from build123d import *

# Parameters (mm, degrees)
F0_W     = 800
F0_H     = 270
F1_DEPTH = 1060
F2_W     = 760
F2_H     = 50
F3_DEPTH = 20
F4_W     = 760
F4_H     = 310
F5_DEPTH = 260


with BuildPart() as f1:
    # F0 (on Top) → F1 (new body)
    with BuildSketch(Plane.XY):
        with Locations((143.156862, -15.404297)):
            Rectangle(F0_W, F0_H)
    extrude(amount=F1_DEPTH)

    # F2 (on face) → F3 (cut)
    with BuildSketch(Plane.XZ.offset(150.404297)):
        with Locations((143.156862, 25)):
            Rectangle(F2_W, F2_H)
    extrude(amount=-F3_DEPTH, mode=Mode.SUBTRACT)

    # F4 (on face) → F5 (cut)
    with BuildSketch(Plane.XZ.offset(150.404297)):
        with Locations((143.156862, 885)):
            Rectangle(F4_W, F4_H)
        with Locations((143.156862, 555)):
            Rectangle(F4_W, F4_H)
        with Locations((143.156862, 225)):
            Rectangle(F4_W, F4_H)
    extrude(amount=-F5_DEPTH, mode=Mode.SUBTRACT)


solid = f1.part
Read the model definition and answer for the solid it produces. Units are mm, in the model's axes. A direction names the side the tool comes from. Coordinates: 2 decimals unless noted, no trailing zeros. Order: outer loops, then holes, each group sorted by start corner. A loop starts at its lowest first (then second) coordinate and runs counter-clockwise, first axis right, second up. Notation, with made-up numbers: (-2, 78) -> (4, 78) arc R38 cw to (4, 116) -> close; hole circle Ø2 at (13.5, 65.5). An arc over 180 degrees is marked (long way). Answer as a JSON object with one key per item and string values.
1) Consider line 1 along Z through (x, y) = (265, -97); line 2 along X through (y, z) = (-49.5, 455); line 3 along Y through (x, z) = (-154, 342). Determine where each line is inside the solid, lowest interval first. Write a range as from..to.
Model answer:
{"line 1": "z = 0..70, 380..400, 710..730, 1040..1060", "line 2": "x = -256.84..-236.84, 523.16..543.16", "line 3": "y = 109.6..119.6"}
2) A tool of negligible diameter and unlimited length cuts with its end or side. For faces 4 (the face through (112, -150.404, 724)), 5 (the face through (138, -130.404, 25)), 6 (the face through (138, 109.596, 227)), from which of +Z, -Z, +X, -X, +Y, -Y can it reach the whole face along a straight path? Write none if from no direction.
Model answer:
{"face 4": "+Z, -Z, +X, -X, -Y", "face 5": "-Z, -Y", "face 6": "-Y"}
3) The mould has two halves that part along Z. Classify faces 1 (the face through (138, -22, 1040)), 2 (the face through (138, 16, 0)), 3 (the face through (543.157, -17, 523)): released by +Z, released by -Z, zero draft, split by the parting line, or undercut.
Model answer:
{"face 1": "undercut", "face 2": "released by -Z", "face 3": "zero draft"}
4) A cutting plane is placed at B-B, the plane y = -95.5. Determine the outline of the cut face in (x, z).
Model answer:
{"outline": "(-256.84, 0) -> (543.16, 0) -> (543.16, 1060) -> (-256.84, 1060) -> close; hole (-236.84, 70) -> (523.16, 70) -> (523.16, 380) -> (-236.84, 380) -> close; hole (-236.84, 400) -> (523.16, 400) -> (523.16, 710) -> (-236.84, 710) -> close; hole (-236.84, 730) -> (523.16, 730) -> (523.16, 1040) -> (-236.84, 1040) -> close"}
5) A cutting plane is placed at C-C, the plane x = -161. Determine the outline of the cut face in (y, z), plus the area to 3 significant figures.
Model answer:
{"outline": "(-150.4, 50) -> (-130.4, 50) -> (-130.4, 0) -> (119.6, 0) -> (119.6, 1060) -> (-150.4, 1060) -> (-150.4, 1040) -> (109.6, 1040) -> (109.6, 730) -> (-150.4, 730) -> (-150.4, 710) -> (109.6, 710) -> (109.6, 400) -> (-150.4, 400) -> (-150.4, 380) -> (109.6, 380) -> (109.6, 70) -> (-150.4, 70) -> close", "area": "43,400 mm²"}
6) Each of these flat-tipped pins is pushed along its axis until it touches: pin 1 (2 mm diameter, centred on x = 126.5, y = 39, fed in from -Z); pin 2 (10 mm diameter, centred on x = 75, y = -140, fed in from -Z); pin 3 (12 mm diameter, centred on x = -111.5, z = 455, fed in from -Y); pin 4 (25 mm diameter, centred on x = 279.5, z = 16.5, fed in from -Y). Where does it stop, or does it pass through?
Model answer:
{"pin 1": "stops at z = 0", "pin 2": "stops at z = 50", "pin 3": "stops at y = 109.6", "pin 4": "stops at y = -130.4"}
7) A cutting plane is placed at A-A, the plane z = 281. Determine the outline of the cut face in (x, y), plus the area to 3 significant figures.
Model answer:
{"outline": "(-256.84, -150.4) -> (-236.84, -150.4) -> (-236.84, 109.6) -> (523.16, 109.6) -> (523.16, -150.4) -> (543.16, -150.4) -> (543.16, 119.6) -> (-256.84, 119.6) -> close", "area": "18,400 mm²"}
